Geometry: final body of the model. Coordinates: model frame, mm. A direction names the side the tool comes from. Give positions to 0.01 mm unless a question says otherwise; leave off trailing zeros. Order: outer loops, then holes, each group sorted by start corner. A loop starts at its lowest first (then second) coordinate and runs counter-clockwise, first axis right, second up. Notation, with made-up numbers: (58.5, -21.5) - (67.5, -21.5) arc R5 cw to (67.5, -16.5) - close; hole circle Ø7 at (38, -19). An arc over 180 degrees is marked (long way). One line per item, written item: value.
```python
from build123d import *

# Parameters (mm, degrees)
SKETCH1_R           = 10
BOSS_EXTRUDE1_DEPTH = 5
SKETCH5_W           = 12.72
SKETCH5_H           = 1.5
CUT_EXTRUDE1_DEPTH  = 20
SKETCH18_R          = 1.5
CUT_EXTRUDE6_DEPTH  = 6
SKETCH10_W          = 3.5
SKETCH10_H          = 20
BOSS_EXTRUDE3_DEPTH = 4.65
SKETCH15_R          = 3
CUT_EXTRUDE4_DEPTH  = 2.5
SKETCH19_R          = 10.05
CUT_EXTRUDE7_DEPTH  = 10.65
BOSS_EXTRUDE6_DEPTH = 4.65
SKETCH24_R          = 1.5
CUT_EXTRUDE8_DEPTH  = 7
SKETCH25_R          = 3
CUT_EXTRUDE9_DEPTH  = 2.5
FILLET5_R           = 3.175


with BuildPart() as part:
    # Sketch1 → Boss-Extrude1 (new body)
    with BuildSketch(Plane.XY):
        with BuildLine():
            Line((9.86, -39), (-9.86, -39))
            Line((-9.86, -39), (-9.86, -16.241317681))
            ThreePointArc((-9.86, -16.241317681), (0, 19), (9.86, -16.241317681))
            Line((9.86, -16.241317681), (9.86, -39))
        make_face()
        Circle(SKETCH1_R, mode=Mode.SUBTRACT)
    extrude(amount=BOSS_EXTRUDE1_DEPTH)

    # Sketch5 → Cut-Extrude1 (cut)
    with BuildSketch(Plane.XZ.offset(39)):
        with Locations((0, 4.25)):
            Rectangle(SKETCH5_W, SKETCH5_H)
    extrude(amount=-CUT_EXTRUDE1_DEPTH, mode=Mode.SUBTRACT)

    # Sketch18 → Cut-Extrude6 (cut, through all)
    with BuildSketch(Plane.XY.offset(5)):
        with Locations((0, -14)):
            Circle(SKETCH18_R)
        with Locations((-12.124355653, 7)):
            Circle(SKETCH18_R)
        with Locations((12.124355653, 7)):
            Circle(SKETCH18_R)
    extrude(amount=-CUT_EXTRUDE6_DEPTH, mode=Mode.SUBTRACT)

    # Sketch10 → Boss-Extrude3 (add)
    with BuildSketch(Plane.XY.offset(5)):
        with Locations((-8.11, -29)):
            Rectangle(SKETCH10_W, SKETCH10_H)
        with Locations((8.11, -29)):
            Rectangle(SKETCH10_W, SKETCH10_H)
    extrude(amount=BOSS_EXTRUDE3_DEPTH)

    # Sketch15 → Cut-Extrude4 (cut)
    with BuildSketch(Plane(origin=(0, 0, 0), x_dir=(-1, 0, 0), z_dir=(0, 0, -1))):
        with Locations((0, -14)):
            Circle(SKETCH15_R)
        with Locations((-12.124355653, 7)):
            Circle(SKETCH15_R)
        with Locations((12.124355653, 7)):
            Circle(SKETCH15_R)
    extrude(amount=-CUT_EXTRUDE4_DEPTH, mode=Mode.SUBTRACT)

    # Sketch19 → Cut-Extrude7 (cut, through all)
    with BuildSketch(Plane(origin=(0, 0, 0), x_dir=(-1, 0, 0), z_dir=(0, 0, -1))):
        Circle(SKETCH19_R)
    extrude(amount=-CUT_EXTRUDE7_DEPTH, mode=Mode.SUBTRACT)

    # Sketch23 → Boss-Extrude6 (add)
    with BuildSketch(Plane.XY.offset(5)):
        with BuildLine():
            Line((9.86, -16.678459911), (9.86, -19))
            Line((9.86, -19), (6.36, -19))
            Line((6.36, -19), (6.36, -18.301394073))
            ThreePointArc((6.36, -18.301394073), (8.150495618, -17.577259348), (9.86, -16.678459911))
        make_face()
    boss_extrude6 = extrude(amount=BOSS_EXTRUDE6_DEPTH)

    # Mirror1: Boss-Extrude6 across plane
    add(boss_extrude6.mirror(Plane(origin=(0, 0, 0), x_dir=(0, 0, 1), z_dir=(1, 0, 0))))

    # Sketch24 → Cut-Extrude8 (cut)
    with BuildSketch(Plane(origin=(0, 0, 0), x_dir=(-1, 0, 0), z_dir=(0, 0, -1))):
        with Locations((0, -31)):
            Circle(SKETCH24_R)
    extrude(amount=-CUT_EXTRUDE8_DEPTH, mode=Mode.SUBTRACT)

    # Sketch25 → Cut-Extrude9 (cut)
    with BuildSketch(Plane(origin=(0, 0, 0), x_dir=(-1, 0, 0), z_dir=(0, 0, -1))):
        with Locations((0, -31)):
            Circle(SKETCH25_R)
    extrude(amount=-CUT_EXTRUDE9_DEPTH, mode=Mode.SUBTRACT)

    # Fillet5
    fillet5_edges = [part.edges().sort_by_distance(p)[0] for p in [
        (9.86, -16.241317681, 2.5),
        (-9.86, -16.241317681, 2.5),
    ]]
    fillet(fillet5_edges, radius=FILLET5_R)


solid = part.part
```
1) Section D-D, the plane z = 7.75. Return loops of the section in (x, y) (3 decimals).
Answers below:
outline: (-10.228, -16.455) arc R3.175 cw to (-9.86, -17.939) - (-9.86, -39) - (-6.36, -39) - (-6.36, -18.301) arc R19.375 cw to start; (6.36, -39) - (9.86, -39) - (9.86, -17.939) arc R3.175 cw to (10.228, -16.455) arc R19.375 cw to (6.36, -18.301) - close
2) Section C-C, the plane x = 12. Return loops of the section in (y, z).
Answers below:
outline: (-14.73, 0) - (4, 0) - (4, 2.5) - (5.51, 2.5) - (5.51, 5) - (-14.73, 5) - close; (8.49, 2.5) - (10, 2.5) - (10, 0) - (14.73, 0) - (14.73, 5) - (8.49, 5) - close
3) Section A-A, the plane z = 1.5. Return loops of the section in (x, y) (3 decimals).
Answers below:
outline: (-11.169, -15.371) arc R3.175 cw to (-9.86, -17.939) - (-9.86, -39) - (9.86, -39) - (9.86, -17.939) arc R3.175 cw to (11.169, -15.371) arc R19 ccw (long way) to start; hole circle Ø6 at (-12.124, 7); hole circle Ø20.1 at (0, 0); hole circle Ø6 at (0, -31); hole circle Ø6 at (0, -14); hole circle Ø6 at (12.124, 7)
4) Mould query, pull axis Y, two halves, no side actions, for faces 4 (the face through (-10.063, -16.821, 3.82)), 5 (the face through (0.65, -33.93, 1.23)), 6 (the face through (-8, -28, 9.65)). Classes: released by +Y, released by -Y, zero draft, split by the parting line, or undercut.
Answers below:
face 4: released by -Y
face 5: undercut
face 6: zero draft
5) Set-up query: faces 1 (the face through (8.318, -17.499, 7.292)), 2 (the face through (6.36, -29, 7)), 3 (the face through (-1.3, -32.3, 2.5)). Return all of +Z, -Z, +X, -X, +Y, -Y with unobstructed straight access to the full face (end or side cutting, diameter ignored); none if empty.
Answers below:
face 1: +Z, +Y
face 2: +Z, -Y
face 3: -Z
6) Section B-B, the plane y = -31. Return loops of the section in (x, z), then the cut area to 3 significant figures.
Answers below:
outline: (-9.86, 0) - (-3, 0) - (-3, 2.5) - (-1.5, 2.5) - (-1.5, 3.5) - (-6.36, 3.5) - (-6.36, 9.65) - (-9.86, 9.65) - close; (1.5, 2.5) - (3, 2.5) - (3, 0) - (9.86, 0) - (9.86, 9.65) - (6.36, 9.65) - (6.36, 3.5) - (1.5, 3.5) - close
area: 94.1 mm^2
7) First-contact query: pin 1 (1.5 mm diameter, centred on x = 11, y = -9.5, fed in from +Z); pin 2 (5.5 mm diameter, centred on x = 0, y = -31, fed in from +Z); pin 3 (1.8 mm diameter, centred on y = -27, z = 8, fed in from +X). Flat tips, straight axial feed; report the tip coordinate or a pass-through.
Answers below:
pin 1: z = 5
pin 2: z = 3.5
pin 3: x = 9.86
8) Material intervals for line 1 along X through (y, z) = (-35.5, 4); line 2 along Z through (x, y) = (-9, -14); line 3 along Y through (x, z) = (-8.5, 3), sorted ascending.
Answers below:
line 1: -9.86 to -6.36, 6.36 to 9.86
line 2: 0 to 5
line 3: -39 to -5.36, 5.36 to 16.99
